The model under review builds one solid part; all positions refer to its coordinate system, in mm. A direction names the side the tool comes from. Round coordinates to 2 decimals unless told otherwise and drop trailing zeros. Order: outer loops, then holes, each group sorted by start corner. A loop starts at its lowest first (then second) coordinate and runs counter-clockwise, first axis right, second up. Notation, with made-up numbers: (-34, 73.25) -> (12, 73.25) arc R5 cw to (12, 78.25) -> close; hole circle Ø8 at (74, 39.25). An arc over 180 degrees is marked (long way). Return JSON: item names as keys, results as strings. Group by question number.
Autodesk Inventor part; units mm, degrees
ref_plane "РабПлоскость1" through (-9.5, 0, 0) normal (1, 0, 0) x (0, 1, 0)
ref_plane "РабПлоскость2" through (0, 0, 12.5) normal (0, 0, -1) x (-1, 0, 0)
ref_plane "РабПлоскость3" through (0, -9.5, 0) normal (0, 1, 0) x (-1, 0, 0)
sketch "Эскиз1" plane through (0, 0, 0) normal (0, 0, 1) x (1, 0, 0)
  circle A0 centre (0, 0) radius 9.5
  dimension "d0" = 19
extrude "Выдавливание1" add sketch "Эскиз1" along normal blind 25
sketch "Эскиз2" plane through (0, 0, 25) normal (0, 0, 1) x (1, 0, 0)
  circle A0 centre (0, 0) radius 3
  dimension "d3" = 6
extrude "Выдавливание2" cut sketch "Эскиз2" against normal blind 12.5
sketch "Эскиз3" plane through (0, 0, 0) normal (0, 0, -1) x (-1, 0, 0)
  circle A0 centre (0, 0) radius 4
  dimension "d6" = 8
extrude "Выдавливание3" cut sketch "Эскиз3" against normal blind 12.5
ref_plane "РабПлоскость1" through (-9.5, 0, 0) normal (1, 0, 0) x (0, 1, 0)
ref_plane "РабПлоскость2" through (0, 0, 12.5) normal (0, 0, -1) x (-1, 0, 0)
sketch "Эскиз5" plane through (0, 0, 12.5) normal (0, 0, -1) x (-1, 0, 0)
  circle A0 centre (0, 0) radius 9.5
  circle A1 centre (0, 0) radius 6.75
  dimension "d20" = 19
  dimension "d21" = 13.5
extrude "Выдавливание5" cut sketch "Эскиз5" along normal mid plane 0.5
pattern_linear "Прямоуг.массив2" count 3 spacing 2 along (0, 0, 1) of "Выдавливание5"
pattern_linear "Прямоуг.массив3" count 3 spacing 2 along (0, 0, -1) of "Выдавливание5"
sketch "Эскиз6" plane through (0, 0, 0) normal (0, 0, -1) x (-1, 0, 0)
  circle A0 centre (0, 0) radius 9.5
  circle A1 centre (0, 0) radius 6.75
  line L0 (-9.5, 0.25) -> (-9.5, 0)
  line L1 (2, 0) -> (2, 0.25)
  line L2 (2, 0.25) -> (-9.5, 0.25)
  line L3 (2, 0) -> (-9.5, 0)
  dimension "d49" = 11.5
  dimension "d50" = 0.25
extrude "Выдавливание6" cut sketch "Эскиз6" against normal up to next contours L0 L2 A0 | A0 L2 A1 L3 | A1 L2 L1 L3 picked at (-7.6653, 0.1389) picked at (-0.9151, 0.1667)
sketch "Эскиз7" plane through (0, 0, 0) normal (0, 0, -1) x (-1, 0, 0)
  arc A0 (-6.75, 0) -> (-6.7454, 0.25) centre (0, 0) ccw
  circle A1 centre (0, 6.75) radius 1
  point P0 (6.7454, 0.25)
  dimension "d33" = 2
extrude "Выдавливание7" cut sketch "Эскиз7" against normal blind 4
pattern_circular "Круговой массив2" count 2 over 360 about axis through (0, 0, 0) along (0, 0, 1) of "Выдавливание7"
mirror "Зеркальное отражение2" about plane through (0, 0, 12.5) normal (0, 0, -1) of "Выдавливание7", "Круговой массив2"
thread "Резьба1"
thread "Резьба2"
thread "Резьба3"
thread "Резьба4"
mirror "Зеркальное отражение3" about plane through (-2, 0, 0) normal (0, 1, 0) of "Выдавливание6"
ref_plane "РабПлоскость3" through (0, -9.5, 0) normal (0, 1, 0) x (-1, 0, 0)
sketch "Эскиз8" plane through (0, -9.5, 0) normal (0, 1, 0) x (-1, 0, 0)
  line L0 (-9.5, -0.0521) -> (-9.5, 3.9479)
  line L1 (-9.5, 3.9479) -> (-7, 3.9479)
  circle A0 centre (-7, 3.9479) radius 1
  point P0 (0, 0)
  dimension "d51" = 2
  dimension "d52" = 2.5
  dimension "d53" = 4
extrude "Выдавливание8" cut sketch "Эскиз8" along normal up to next
sketch "Эскиз9" plane through (0, -9.5, 0) normal (0, 1, 0) x (-1, 0, 0)
  circle A0 centre (-7, 3.9479) radius 1
  circle A1 centre (-7, 3.9479) radius 2
  point P0 (0, 0)
  dimension "d56" = 4
extrude "Выдавливание9" cut sketch "Эскиз9" along normal blind 5
ref_plane "РабПлоскость5" through (0, 9.5, 0) normal (0, 1, 0) x (-1, 0, 0)
sketch "Эскиз10" plane through (0, 9.5, 0) normal (0, 1, 0) x (-1, 0, 0)
  circle A0 centre (-7, 3.9479) radius 1
  circle A1 centre (-7, 3.9479) radius 1
  point P0 (0, 0)
extrude "Выдавливание10" cut sketch "Эскиз10" against normal up to next
sketch "Эскиз11" plane through (0, 9.5, 0) normal (0, 1, 0) x (-1, 0, 0)
  circle A0 centre (-7, 3.9479) radius 1
  circle A1 centre (-7, 3.9479) radius 2
  point P0 (0, 0)
extrude "Выдавливание11" cut sketch "Эскиз11" against normal blind 5
mirror "Зеркальное отражение10" about plane through (0, 0, 12.5) normal (0, 0, -1) of "Выдавливание8", "Выдавливание9"
mirror "Зеркальное отражение11" about plane through (0, 0, 12.5) normal (0, 0, -1) of "Выдавливание10", "Выдавливание11"
properties part number "Муфта4х5"
Item 1: For faces 5 (the face through (0, 7, 21)), 6 (the face through (6, 0.25, 12)), 7 (the face through (0, -7, 4)), 8 (the face through (-4, -6, 10.25)), 9 (the face through (5, -6, 4)), list the 3-axis set-ups (+Z, -Z, +X, -X, +Y, -Y) from which the entire face can be reached by the end or side of a thin tool; tool diameter is ignored.
Item 2: The part is to be moulded in two halves that separate along Y. For faces 1 (the face through (1, -3, 12.5)), 2 (the face through (-4, -6, 12.75)), 3 (the face through (-6.744, 0.293, 8.504)), 4 (the face through (6, 4.5, 5)), say which applies: +Y half, -Y half, draft (parallel to the pull), parting line (faces both ways), or undercut.
Item 3: Consider section A-A on z = 21.5. State the section outline as (x, y) points.
Item 4: Wall thickness on line 1 along Z through (x, y) = (4.75, 7.25); line 2 along Y through (x, z) = (0, 24.25); line 3 along Z through (x, y) = (0.25, -7): over which ranges is each line inside the solid? List them lowest first.
Item 5: Consider section B-B on y = -2. Give the number of separate pieces and of enclosed holes in the cut face, plus the area to 3 significant figures.
Item 6: Insertion check: pin 1 Ø2.5 at (x, z) = (6.5, 5) entering from -Y; pin 2 Ø2 at (x, z) = (7.5, 10.5) entering from +Y; pin 3 Ø5.5 at (x, y) = (-2.5, 0) entering from -Z; pin 4 Ø1.2 at (x, y) = (0, -6.75) entering from -Z. Each pin has a flat end and moves straight along its axis. Give the tip position at first contact, or say it passes through.
Values:
{
 "1": {"face 5": "+Z", "face 6": "+Z, -Z, +X", "face 7": "-Z", "face 8": "none", "face 9": "-Y"},
 "2": {"face 1": "undercut", "face 2": "draft", "face 3": "parting line", "face 4": "+Y half"},
 "3": {"outline": "(2.99, -0.25) arc R3 cw (long way) to (2.99, 0.25) -> (6.11, 0.25) -> (6.11, 4.5) -> (5.05, 4.5) -> (5.05, 8.05) arc R9.5 ccw (long way) to (5.05, -8.05) -> (5.05, -4.5) -> (6.11, -4.5) -> (6.11, -0.25) -> close; (7.89, -4.5) -> (8.37, -4.5) arc R9.5 ccw to (9.5, -0.25) -> (7.89, -0.25) -> close; (7.89, 0.25) -> (9.5, 0.25) arc R9.5 ccw to (8.37, 4.5) -> (7.89, 4.5) -> close; hole circle Ø2 at (0, -6.75); hole circle Ø2 at (0, 6.75)"},
 "4": {"line 1": "0 to 8.25, 8.75 to 10.25, 10.75 to 12.25, 12.75 to 14.25, 14.75 to 16.25, 16.75 to 25", "line 2": "-9.5 to -7.75, -5.75 to -3, 3 to 5.75, 7.75 to 9.5", "line 3": "4 to 8.25, 8.75 to 10.25, 10.75 to 12.25, 12.75 to 14.25, 14.75 to 16.25, 16.75 to 21"},
 "5": {"separate pieces": "2", "enclosed holes": "2", "area": "301 mm^2"},
 "6": {"pin 1": "y = -7.92", "pin 2": "y = 6.9", "pin 3": "z = 0", "pin 4": "z = 4"}
}
